Autodesk Inventor part; units mm, degrees
ref_plane "YZ Plane" through (0, 0, 0) normal (1, 0, 0) x (0, 1, 0)
ref_plane "XZ Plane" through (0, 0, 0) normal (0, 1, 0) x (-1, 0, 0)
ref_plane "XY Plane" through (0, 0, 0) normal (0, 0, 1) x (1, 0, 0)
sketch "スケッチ1" plane through (0, 0, 0) normal (0, 0, 1) x (1, 0, 0)
  line L0 (0, 0) -> (110, 0)
  line L1 (110, 0) -> (110, 10)
  line L2 (110, 10) -> (55, 10)
  line L3 (55, 10) -> (55, 31)
  line L4 (55, 31) -> (45, 31)
  line L5 (45, 31) -> (45, 10)
  line L6 (45, 10) -> (0, 10)
  line L7 (0, 10) -> (0, 0)
  dimension "d0" = 110
  dimension "d1" = 10
  dimension "d2" = 21
  dimension "d3" = 10
  dimension "d4" = 45
extrude "押し出し1" add sketch "スケッチ1" along normal blind 20
sketch "スケッチ2" plane through (0, 0, 0) normal (0, -1, 0) x (1, 0, 0)
  line L0 (110, 0) -> (110, 20) construction
  line L1 (110, 10) -> (0, 10) construction
  line L2 (0, 0) -> (0, 20) construction
  circle A0 centre (100, 10) radius 2.75
  circle A1 centre (10, 10) radius 2.75
  line L3 (0, 0) -> (110, 0) construction
  line L4 (55, 0) -> (55, 20) construction
  line L5 (0, 20) -> (110, 20) construction
  circle A2 centre (80, 10) radius 1.75
  circle A3 centre (30, 10) radius 1.75
  dimension "d7" = 5.5
  dimension "d8" = 10
  dimension "d9" = 10
  dimension "d17" = 3.5
  dimension "d18" = 50
extrude "押し出し2" cut sketch "スケッチ2" against normal through all
sketch "スケッチ3" plane through (45, 10, 0) normal (-1, 0, 0) x (0, 0, 1)
  line L0 (0, 21) -> (20, 21) construction
  line L1 (10, 21) -> (10, 0) construction
  line L2 (0, 0) -> (20, 0) construction
  circle A0 centre (10, 11) radius 2.75
  point P0 (0, -10)
  dimension "d12" = 10
  dimension "d13" = 5.5
extrude "押し出し3" cut sketch "スケッチ3" against normal through all
fillet "フィレット1" radius 10 2 edges at (50, 31, 0) (50, 31, 20)
fillet "フィレット2" radius 2 4 edges at (110, 5, 20) (110, 5, 0) (0, 5, 0) (0, 5, 20)
properties part number "_3D プリント"
CAD build for the part. Positions are in the model's coordinates, mm. A direction names the side the tool comes from. Round coordinates to 2 decimals unless told otherwise and drop trailing zeros. Write each loop counter-clockwise with the first axis right and the second up, starting at its lowest first coordinate (ties: lowest second). Pieces come first, ordered by that corner, then holes. Notation, with made-up numbers: (62, 48) -> (77, 48) arc R27 cw to (77, 87) -> close; hole circle Ø8 at (10.25, 28). An arc over 180 degrees is marked (long way). Answer in a Markdown table with one row per item. Add a question column.
Item 1: Which spindle directions (+Z, -Z, +X, -X, +Y, -Y) get a long thin tool onto all of the face, cutting with end or side? Do faces 1 (the face through (45, 18, 12)), 2 (the face through (83, 10, 10)), 3 (the face through (110, 5, 10)). Say none if no direction does.
Item 2: Mould opens along Z. For faces 4 (the face through (11.48, 4.93, 12.32)), 5 (the face through (0.6, 4.93, 19.43)), 6 (the face through (49.93, 28.15, 3.01)), 7 (the face through (28.25, 4.93, 10.08)) say: pulls with the +Z half, pulls with the -Z half, needs draft (parallel to the pull), parting line crosses it, or undercut.
Item 3: Saw through at A-A, the plane x = 100. Write the cut outline in (y, z).
Item 4: Drop flat-ended pins along their axis: pin 1 Ø5 at (y, z) = (16, 17) entering from -X; pin 2 Ø6 at (x, z) = (40, 11) entering from +Y; pin 3 Ø1 at (y, z) = (24, 8) entering from +X. Give the stop position or say it passes through.
Item 5: Drill centre lines: line 1 (Z direction, x = 100, y = 4); line 2 (Y direction, x = 50.5, z = 10); line 3 (Y direction, x = 5, z = 4.5). Where is each one in solid material? Low to high. Write a range as from..to.
Item 6: Saw through at C-C, the plane x = 30. Write the cut outline in (y, z), then the cut area to 3 significant figures.
Item 7: Saw through at D-D, the plane y = 12. Write the cut outline in (x, z), then the cut area to 3 significant figures.
Item 8: Saw through at B-B, the plane z = 16.5. Write the cut outline in (x, y).
Findings below:
| question | item | result |
|---|---|---|
| 1 | face 1 | +Z, -Z, -X, +Y |
| 1 | face 2 | +Z, -Z, +X, +Y |
| 1 | face 3 | +Z, -Z, +X, +Y, -Y |
| 2 | face 4 | undercut |
| 2 | face 5 | pulls with the +Z half |
| 2 | face 6 | pulls with the -Z half |
| 2 | face 7 | undercut |
| 3 | outline | (0, 0) -> (10, 0) -> (10, 7.25) -> (0, 7.25) -> close; (0, 12.75) -> (10, 12.75) -> (10, 20) -> (0, 20) -> close |
| 4 | pin 1 | stops at x = 45 |
| 4 | pin 2 | stops at y = 10 |
| 4 | pin 3 | stops at x = 55 |
| 5 | line 1 | z = 0..7.25, 12.75..20 |
| 5 | line 2 | y = 0..18.25, 23.75..31 |
| 5 | line 3 | y = 0..10 |
| 6 | outline | (0, 0) -> (10, 0) -> (10, 8.25) -> (0, 8.25) -> close; (0, 11.75) -> (10, 11.75) -> (10, 20) -> (0, 20) -> close |
| 6 | area | 165 mm^2 |
| 7 | outline | (45, 0) -> (55, 0) -> (55, 20) -> (45, 20) -> close |
| 7 | area | 200 mm^2 |
| 8 | outline | (0, 0) -> (110, 0) -> (110, 10) -> (55, 10) -> (55, 28.6) -> (45, 28.6) -> (45, 10) -> (0, 10) -> close |
